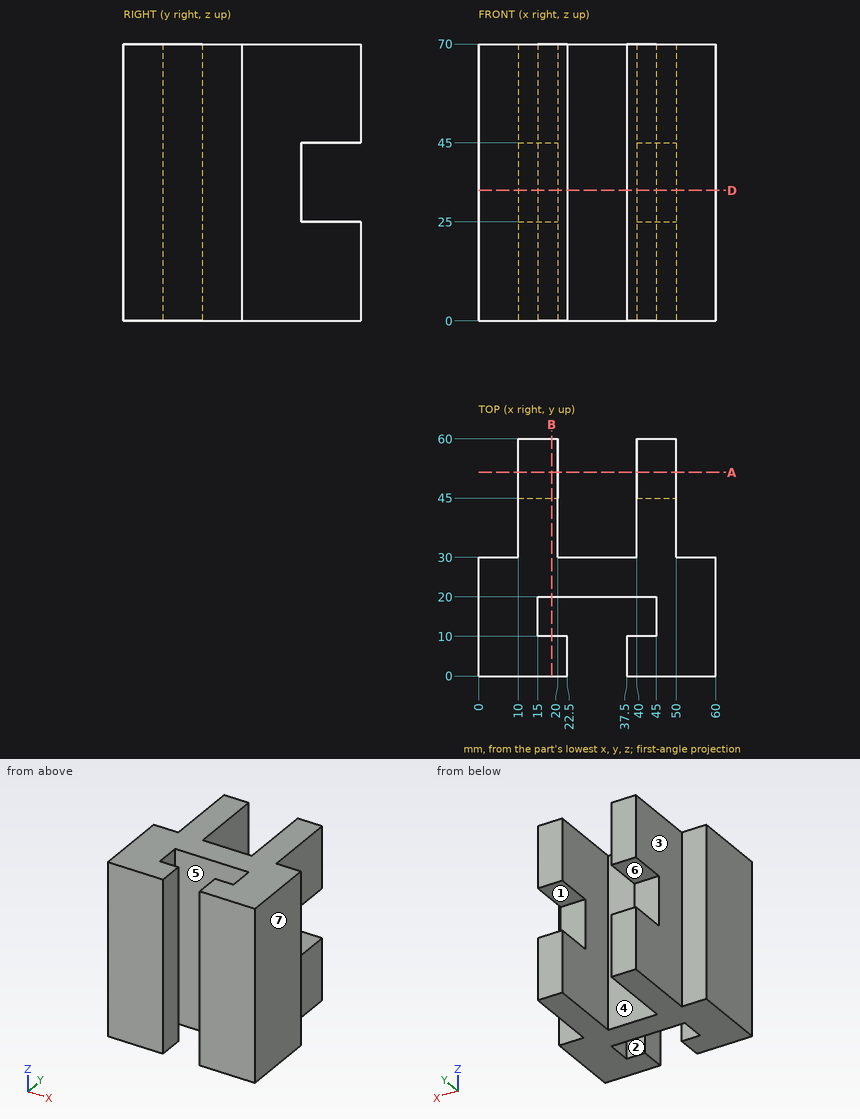
Study the drawing (mm; zero at the part's minimum x, y, z) and answer. A direction names the side the tool comes from. Coordinates: 2 decimals unless noted, no trailing zeros. Write each loop counter-clockwise with the first axis right and the second up, starting at its lowest first coordinate (ties: lowest second). Pieces come first, ordered by that corner, then holes. Notation, with made-up numbers: (23.25, -5) - (69.25, -5) arc R26 ccw to (69.25, 29) - close; hole circle Ø3 at (54.25, 54.25). An arc over 180 degrees is marked (long way). Answer as a JSON object with one key per item and string values. Group by question number.
1. Consider L1, parallel to X at y = 42, z = 47; L2, parallel to X at y = 8, z = 58; L3, parallel to Z at x = 19, y = 47.5. Determine where each line is inside the solid, lowest interval first. Write a range as [from, to].
2. Each of these flat-tipped pins is pushed along its axis until it touches: P1, Ø8, axis at x = 47.5, z = 35, coming from the +Y side; P2, Ø1, axis at x = 32.5, z = 9, coming from the +Y side; P3, Ø5, axis at x = 34, z = 27.5, coming from the -Y side. Where does it stop, or does it pass through?
3. A cutting plane is placed at A-A (y = 51.5). Determine the outline of the cut face in (x, z).
4. A cutting plane is placed at B-B (x = 18.5). Determine the outline of the cut face in (y, z).
5. Which of the six approach directions +Z, -Z, +X, -X, +Y, -Y give full straight-line access (tool end or side, diameter ignored) to the marked faces 1, 2, 3 and 4?
6. A cutting plane is placed at D-D (z = 33). Determine the outline of the cut face in (x, y).
7. The mould has two halves that part along X. Classify the marked faces 5, 6 and 7: +X half, -X half, draft (parallel to the pull), parting line (faces both ways), or undercut.
Worked out:
{
 "1": {"L1": "x = [10, 20], [40, 50]", "L2": "x = [0, 22.5], [37.5, 60]", "L3": "z = [0, 25], [45, 70]"},
 "2": {"P1": "stops at y = 45", "P2": "stops at y = 30", "P3": "stops at y = 20"},
 "3": {"outline": "(10, 0) - (20, 0) - (20, 25) - (10, 25) - close; (10, 45) - (20, 45) - (20, 70) - (10, 70) - close; (40, 0) - (50, 0) - (50, 25) - (40, 25) - close; (40, 45) - (50, 45) - (50, 70) - (40, 70) - close"},
 "4": {"outline": "(0, 0) - (10, 0) - (10, 70) - (0, 70) - close; (20, 0) - (60, 0) - (60, 25) - (45, 25) - (45, 45) - (60, 45) - (60, 70) - (20, 70) - close"},
 "5": {"face 1": "+X, -X, +Y", "face 2": "+Z, -Z", "face 3": "+Z, -Z, -X, +Y", "face 4": "+Z, -Z, +Y"},
 "6": {"outline": "(0, 0) - (22.5, 0) - (22.5, 10) - (15, 10) - (15, 20) - (45, 20) - (45, 10) - (37.5, 10) - (37.5, 0) - (60, 0) - (60, 30) - (50, 30) - (50, 45) - (40, 45) - (40, 30) - (20, 30) - (20, 45) - (10, 45) - (10, 30) - (0, 30) - close"},
 "7": {"face 5": "undercut", "face 6": "draft", "face 7": "+X half"}
}
